Work out the finished part from the listing and answer in its coordinate system (mm). Face numbers are marked on the shaded views. A direction names the side the tool comes from. Give positions to 0.01 mm unless a question says otherwise; leave off trailing zeros. Put each result on its own line as item: value.
```python
from build123d import *
from OCP.BRepAlgoAPI import BRepAlgoAPI_Cut
from OCP.TopTools import TopTools_ListOfShape

# Parameters (mm, degrees)
SKETCH4_R               = 2.235
SKETCH3_R               = 2.31
CUT_EXTRUDE1_DEPTH      = 27.58647073088115
CUT_EXTRUDE1_DEPTH_BACK = 27.58647073088115
BOSS_EXTRUDE1_DEPTH     = 0.72
CUT_EXTRUDE2_DEPTH      = 27.578153590375337
CUT_EXTRUDE2_DEPTH_BACK = 27.578153590375337
SKETCH11_R              = 0.5000000000000008
CUT_EXTRUDE3_DEPTH      = 27.578153590375337
CUT_EXTRUDE3_DEPTH_BACK = 27.578153590375337
CUT_EXTRUDE4_DEPTH      = 27.578153590375337
CUT_EXTRUDE4_DEPTH_BACK = 27.578153590375337


with BuildPart() as part:
    # Sketch4 → Loft1 section 0
    with BuildSketch(Plane.XY.offset(10.64)):
        Circle(SKETCH4_R)
    # Sketch3 → Loft1 section 1
    with BuildSketch(Plane.XY):
        Circle(SKETCH3_R)
    loft()

    # Loft2: read off the stored shape, not the designer's step
    # Loft2: loft between two sections, ruled curve by curve
    loft2_from = [
        Edge.make_bspline([(-1.907298859, 0.260453572, 10.64), (-2.428206003, -3.554144145, 10.64), (1.386391714, -4.07505129, 10.64), (1.907298859, -0.260453572, 10.64), (2.428206003, 3.554144145, 10.64), (-1.386391714, 4.07505129, 10.64), (-1.907298859, 0.260453572, 10.64)], [0, 0, 0, 0, 0.5, 0.5, 0.5, 1, 1, 1, 1], 3, [1, 0.333333333333333, 0.333333333333333, 1, 0.333333333333333, 0.333333333333333, 1]),
    ]
    loft2_to = [
        Edge.make_bspline([(-0.608448322, 0.557149567, 25.56), (-1.722747455, -0.659747077, 25.56), (-0.505850812, -1.77404621, 25.56), (0.608448322, -0.557149567, 25.56), (1.722747455, 0.659747077, 25.56), (0.505850812, 1.77404621, 25.56), (-0.608448322, 0.557149567, 25.56)], [0, 0, 0, 0, 0.5, 0.5, 0.5, 1, 1, 1, 1], 3, [1, 0.333333333333333, 0.333333333333333, 1, 0.333333333333333, 0.333333333333333, 1]),
    ]
    loft2 = Solid(Shell([*[Face.make_surface_from_curves(loft2_from[k], loft2_to[k]) for k in range(1)], Face(Wire(loft2_from)), Face(Wire(loft2_to))]))
    add(loft2)

    # Revolve3: read off the stored shape, not the designer's step
    # Revolve3 outline → Revolve3 (revolve)
    with BuildSketch(Plane.XZ):
        with BuildLine():
            Line((0, 25.56), (0.825, 25.56))
            ThreePointArc((0.825, 25.56), (0.583363094, 26.143363094), (0, 26.385))
            Line((0, 26.385), (0, 25.56))
        make_face()
    revolve(axis=Axis((0, 0, 0), (0, 0, 1)))


with BuildPart() as cut_extrude1_tool:
    # Sketch9 → Cut-Extrude1 (new, two sides: drawn at the far end of the back side and taken through both)
    with BuildSketch(Plane(origin=(0, 0, 0), x_dir=(0, 0, -1), z_dir=(1, 0, 0)).offset(-CUT_EXTRUDE1_DEPTH_BACK)):
        with BuildLine():
            Line((0, 2.31), (-5.74, 2.269539473684211))
            ThreePointArc((-5.74, 2.269539473684211), (-7.993598162174239, -2.37e-14), (-5.74, -2.2695394736842105))
            Line((-5.74, -2.2695394736842105), (0, -2.31))
            Line((0, -2.31), (0, 2.31))
        make_face()
    extrude(amount=CUT_EXTRUDE1_DEPTH + CUT_EXTRUDE1_DEPTH_BACK)


with BuildPart() as part_1:
    add(part.part)

    # Cut-Extrude1: cut by cut_extrude1_tool, with a tolerance
    cut_extrude1_stock = TopTools_ListOfShape()
    cut_extrude1_stock.Append(part_1.part.wrapped)
    cut_extrude1_tools = TopTools_ListOfShape()
    cut_extrude1_tools.Append(cut_extrude1_tool.part.wrapped)
    cut_extrude1_cut = BRepAlgoAPI_Cut()
    cut_extrude1_cut.SetArguments(cut_extrude1_stock)
    cut_extrude1_cut.SetTools(cut_extrude1_tools)
    cut_extrude1_cut.SetFuzzyValue(0.00001)
    cut_extrude1_cut.Build()
    add(Compound.cast(cut_extrude1_cut.Shape()).solids(), mode=Mode.REPLACE)

    # Sketch10 → Boss-Extrude1 (add)
    with BuildSketch(Plane(origin=(0, 0, 0), x_dir=(0, 0, -1), z_dir=(1, 0, 0))):
        with BuildLine():
            Line((-5.755997693658497, 2.2695958558327507), (-1.515997693658497, 2.2695958558327507))
            ThreePointArc((-1.515997693658497, 2.2695958558327507), (-0.01599769365849646, 0.769595855832751), (-1.5159976936584965, -0.7304041441672493))
            Line((-1.5159976936584965, -0.7304041441672493), (-5.755997693658497, -0.7304041441672493))
            ThreePointArc((-5.755997693658497, -0.7304041441672493), (-6.300456135431979, -0.5691848113978423), (-6.754869150888661, -0.22869181666727964))
            ThreePointArc((-6.754869150888661, -0.22869181666727964), (-7.3637940337605725, -0.01339161533026489), (-8.009638140649475, -0.0079990952139372))
            ThreePointArc((-8.009638140649475, -0.0079990952139372), (-7.353348220945002, 1.5963799024633214), (-5.755997693658497, 2.2695958558327507))
        make_face()
    extrude(amount=-BOSS_EXTRUDE1_DEPTH)

    # Sketch11 → Cut-Extrude2 (cut, two sides: drawn at the far end of the back side and taken through both)
    with BuildSketch(Plane(origin=(0, 0, 0), x_dir=(0, 0, -1), z_dir=(1, 0, 0)).offset(-CUT_EXTRUDE2_DEPTH_BACK)):
        with Locations(Location((-5.755997693658496, -0.08040414416724939, 0), (0, 0, 179.999999999))):
            Circle(SKETCH11_R)
    extrude(amount=CUT_EXTRUDE2_DEPTH + CUT_EXTRUDE2_DEPTH_BACK, mode=Mode.SUBTRACT)

    # Sketch12 → Cut-Extrude3 (cut, two sides: drawn at the far end of the back side and taken through both)
    with BuildSketch(Plane(origin=(0, 0, 0), x_dir=(0, 0, -1), z_dir=(1, 0, 0)).offset(-CUT_EXTRUDE3_DEPTH_BACK)):
        with BuildLine():
            Line((-2.61955108425177, -0.4339575347605234), (-3.326657865438317, 0.2731492464260242))
            ThreePointArc((-3.326657865438317, 0.2731492464260242), (-3.3266578654383174, 0.980256027612572), (-2.6195510842517695, 0.9802560276125718))
            Line((-2.6195510842517695, 0.9802560276125718), (-1.9124443030652216, 0.27314924642602484))
            ThreePointArc((-1.9124443030652216, 0.27314924642602484), (-1.9124443030652214, -0.43395753476052357), (-2.61955108425177, -0.4339575347605234))
        make_face()
    extrude(amount=CUT_EXTRUDE3_DEPTH + CUT_EXTRUDE3_DEPTH_BACK, mode=Mode.SUBTRACT)

    # Sketch8 → Cut-Extrude4 (cut, two sides: drawn at the far end of the back side and taken through both)
    with BuildSketch(Plane(origin=(0, 0, 0), x_dir=(0, 0, -1), z_dir=(1, 0, 0)).offset(-CUT_EXTRUDE4_DEPTH_BACK)):
        Polygon((-10.64, 4.3e-16), (-10.92678821817553, 0.4095760221444918), (-11.500364653175215, -0.40957602021520884), (-12.073941088175136, 0.40957602214423094), (-12.647517523174814, -0.40957602021521683), (-13.221093958174729, 0.40957602214440114), (-13.794670393174655, -0.40957602021506484), (-14.368246828174327, 0.4095760221443932), (-14.941823263174012, -0.409576020215047), (-15.515399698173928, 0.40957602214438515), (-16.088976133173613, -0.409576020215055), (-16.662552568173783, 0.40957602214437716), (-17.236129003173215, -0.4095760202152489), (-17.809705438173125, 0.4095760221443691), (-18.38328187317281, -0.40957602021507106), (-18.956858308172723, 0.4095760221443611), (-19.53043474317241, -0.40957602021507905), (-20.10401117817232, 0.4095760221443531), (-20.67758761317201, -0.4095760202150871), (-21.25116404817192, 0.4095760221443451), (-21.82474048317161, -0.4095760202150951), (-22.398316918171524, 0.4095760221443371), (-22.971893353171208, -0.40957602021510314), (-23.545469788171122, 0.4095760221443291), (-24.119046223170805, -0.4095760202151111), (-24.69262265817072, 0.4095760221443211), (-25.266199093170407, -0.40957602021511913), (-25.839775528170343, 0.4095760221440387), (-26.413351963170005, -0.4095760202151271), (-26.986928398169923, 0.40957602214430294), (-26.986928398169923, -4.419260588317123), (-4.451704701186554, -4.419260588317123), (-4.451704701186554, -2.80017242629016), (-7.993591564895423, -0.00547231851227717), align=None)
    extrude(amount=CUT_EXTRUDE4_DEPTH + CUT_EXTRUDE4_DEPTH_BACK, mode=Mode.SUBTRACT)


solid = part_1.part
```
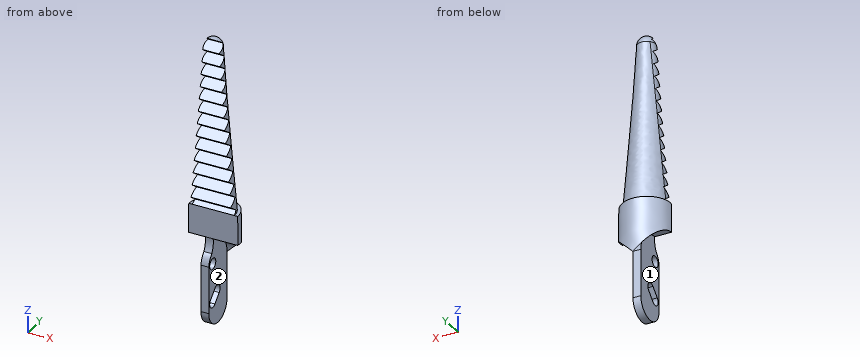
(1) Straight lines are drawn through the part: line 1 (X direction, y = 2.1, z = 1.75); line 2 (X direction, y = 0.15, z = 10); line 3 (Y direction, x = 0.75, z = 11.25). For each, find the intervals that lie inside material, in ascending order.
Geometry check:
line 1: x = -0.72 to 0
line 2: x = -2.23 to 2.23
line 3: y = -0.05 to 1.72
(2) A tool of negligible diameter and unlimited length cuts with its end or side. For the marked faces 1 and 2, from which of +Z, -Z, +X, -X, +Y, -Y can it reach the whole face along a straight path? Write none if from no direction.
Geometry check:
face 1: -Z, -X, -Y
face 2: -Z, +X, -Y
(3) Given pin 1 (1 mm diameter, centred on y = 0.5, z = 19, fed in from +X); pin 2 (1.5 mm diameter, centred on y = 0, z = 3, fed in from -X); pin 3 (1.6 mm diameter, centred on y = -0.08, z = 5.76, fed in from +X), each flat-ended and moving along its own axis, determine where each tip first touches the part or whether it passes through.
Geometry check:
pin 1: stops at x = 1.27
pin 2: stops at x = -0.72
pin 3: stops at x = 0
